from build123d import *

# Parameters (mm, degrees)
SKETCH_1_R          = 1.6
SKETCH_1_R_2        = 3.05
SKETCH_1_W          = 1.5
SKETCH_1_H          = 1.949874371
EXTRUDE_1_DEPTH     = 11
SKETCH_2_R          = 1.65
CUT_EXTRUDE_3_DEPTH = 21.223748416


with BuildPart() as part:
    # Sketch 1 → Extrude 1 (new body)
    # profile 1 of 23: a face of its own
    with BuildSketch(Plane.XY):
        with BuildLine():
            Line((-0.75, 9.971835338), (-0.75, 12))
            Line((-0.75, 12), (-1, 9.949874371))
            ThreePointArc((-1, 9.949874371), (-0.875068895, 9.961639144), (-0.75, 9.971835338))
        make_face()
    # profile 2 of 23: a face of its own
    with BuildSketch(Plane.XY):
        with BuildLine():
            Line((0.75, 12), (-0.75, 12))
            Line((-0.75, 12), (-0.75, 9.971835338))
            ThreePointArc((-0.75, 9.971835338), (0, 10), (0.75, 9.971835338))
            Line((0.75, 9.971835338), (0.75, 12))
        make_face()
    # profile 3 of 23: a face of its own
    with BuildSketch(Plane.XY):
        with BuildLine():
            ThreePointArc((-0.75, 9.971835338), (-0.875068895, 9.961639144), (-1, 9.949874371))
            Line((-1, 9.949874371), (-0.75, 9.949874371))
            Line((-0.75, 9.949874371), (-0.75, 9.971835338))
        make_face()
    # profile 4 of 23: a face of its own
    with BuildSketch(Plane.XY):
        with BuildLine():
            Line((-0.75, 9.949874371), (-1, 9.949874371))
            ThreePointArc((-1, 9.949874371), (-1.95090322, 9.807852804), (-2.883772543, 9.575168715))
            ThreePointArc((-2.883772543, 9.575168715), (-3.826834324, 9.238795325), (-4.731531608, 8.80980185))
            ThreePointArc((-4.731531608, 8.80980185), (-5.55570233, 8.314696123), (-6.328516859, 7.742730421))
            ThreePointArc((-6.328516859, 7.742730421), (-7.071067812, 7.071067812), (-7.742730421, 6.328516859))
            ThreePointArc((-7.742730421, 6.328516859), (-8.314696123, 5.55570233), (-8.80980185, 4.731531608))
            ThreePointArc((-8.80980185, 4.731531608), (-9.238795325, 3.826834324), (-9.575168715, 2.883772543))
            ThreePointArc((-9.575168715, 2.883772543), (-9.807852804, 1.95090322), (-9.949874371, 1))
            ThreePointArc((-9.949874371, 1), (-10, 0), (-9.949874371, -1))
            ThreePointArc((-9.949874371, -1), (-9.807852804, -1.95090322), (-9.575168715, -2.883772543))
            ThreePointArc((-9.575168715, -2.883772543), (-9.238795325, -3.826834324), (-8.80980185, -4.731531608))
            ThreePointArc((-8.80980185, -4.731531608), (-8.314696123, -5.55570233), (-7.742730421, -6.328516859))
            ThreePointArc((-7.742730421, -6.328516859), (-7.071067812, -7.071067812), (-6.328516859, -7.742730421))
            ThreePointArc((-6.328516859, -7.742730421), (-5.55570233, -8.314696123), (-4.731531608, -8.80980185))
            ThreePointArc((-4.731531608, -8.80980185), (-3.826834324, -9.238795325), (-2.883772543, -9.575168715))
            ThreePointArc((-2.883772543, -9.575168715), (-1.95090322, -9.807852804), (-1, -9.949874371))
            ThreePointArc((-1, -9.949874371), (0, -10), (1, -9.949874371))
            ThreePointArc((1, -9.949874371), (1.95090322, -9.807852804), (2.883772543, -9.575168715))
            ThreePointArc((2.883772543, -9.575168715), (3.826834324, -9.238795325), (4.731531608, -8.80980185))
            ThreePointArc((4.731531608, -8.80980185), (5.55570233, -8.314696123), (6.328516859, -7.742730421))
            ThreePointArc((6.328516859, -7.742730421), (7.071067812, -7.071067812), (7.742730421, -6.328516859))
            ThreePointArc((7.742730421, -6.328516859), (8.314696123, -5.55570233), (8.80980185, -4.731531608))
            ThreePointArc((8.80980185, -4.731531608), (9.238795325, -3.826834324), (9.575168715, -2.883772543))
            ThreePointArc((9.575168715, -2.883772543), (9.807852804, -1.95090322), (9.949874371, -1))
            ThreePointArc((9.949874371, -1), (9.987460731, -0.500627751), (10, 0))
            ThreePointArc((10, 0), (9.987460731, 0.500627751), (9.949874371, 1))
            ThreePointArc((9.949874371, 1), (9.807852804, 1.95090322), (9.575168715, 2.883772543))
            ThreePointArc((9.575168715, 2.883772543), (9.238795325, 3.826834324), (8.80980185, 4.731531608))
            ThreePointArc((8.80980185, 4.731531608), (8.314696123, 5.55570233), (7.742730421, 6.328516859))
            ThreePointArc((7.742730421, 6.328516859), (7.071067812, 7.071067812), (6.328516859, 7.742730421))
            ThreePointArc((6.328516859, 7.742730421), (5.55570233, 8.314696123), (4.731531608, 8.80980185))
            ThreePointArc((4.731531608, 8.80980185), (3.826834324, 9.238795325), (2.883772543, 9.575168715))
            ThreePointArc((2.883772543, 9.575168715), (1.95090322, 9.807852804), (1, 9.949874371))
            Line((1, 9.949874371), (0.75, 9.949874371))
            Line((0.75, 9.949874371), (0.75, 8))
            Line((0.75, 8), (-0.75, 8))
            Line((-0.75, 8), (-0.75, 9.949874371))
        make_face()
        with Locations((0, -6.363961031)):
            Circle(SKETCH_1_R, mode=Mode.SUBTRACT)
        with Locations((-6.363961031, 0)):
            Circle(SKETCH_1_R, mode=Mode.SUBTRACT)
        Circle(SKETCH_1_R_2, mode=Mode.SUBTRACT)
        with Locations((6.363961031, 0)):
            Circle(SKETCH_1_R, mode=Mode.SUBTRACT)
        with Locations((0, 6.363961031)):
            Circle(SKETCH_1_R, mode=Mode.SUBTRACT)
    # profile 5 of 23: a face of its own
    with BuildSketch(Plane.XY):
        with BuildLine():
            Line((1, 9.949874371), (0.75, 12))
            Line((0.75, 12), (0.75, 9.971835338))
            ThreePointArc((0.75, 9.971835338), (0.875068895, 9.961639144), (1, 9.949874371))
        make_face()
    # profile 6 of 23: a face of its own
    with BuildSketch(Plane.XY):
        with BuildLine():
            ThreePointArc((0.75, 9.971835338), (0, 10), (-0.75, 9.971835338))
            Line((-0.75, 9.971835338), (-0.75, 9.949874371))
            Line((-0.75, 9.949874371), (0.75, 9.949874371))
            Line((0.75, 9.949874371), (0.75, 9.971835338))
        make_face()
    # profile 7 of 23: a face of its own
    with BuildSketch(Plane.XY):
        with Locations((0, 8.974937185)):
            Rectangle(SKETCH_1_W, SKETCH_1_H)
    # profile 8 of 23: a face of its own
    with BuildSketch(Plane.XY):
        with BuildLine():
            ThreePointArc((-4.731531608, 8.80980185), (-3.826834324, 9.238795325), (-2.883772543, 9.575168715))
            Line((-2.883772543, 9.575168715), (-3.899291539, 11.373566964))
            Line((-3.899291539, 11.373566964), (-5.285110838, 10.799541816))
            Line((-5.285110838, 10.799541816), (-4.731531608, 8.80980185))
        make_face()
    # profile 9 of 23: a face of its own
    with BuildSketch(Plane.XY):
        with BuildLine():
            ThreePointArc((1, 9.949874371), (0.875068895, 9.961639144), (0.75, 9.971835338))
            Line((0.75, 9.971835338), (0.75, 9.949874371))
            Line((0.75, 9.949874371), (1, 9.949874371))
        make_face()
    # profile 10 of 23: a face of its own
    with BuildSketch(Plane.XY):
        with BuildLine():
            Line((3.899291539, 11.373566964), (2.883772543, 9.575168715))
            ThreePointArc((2.883772543, 9.575168715), (3.826834324, 9.238795325), (4.731531608, 8.80980185))
            Line((4.731531608, 8.80980185), (5.285110838, 10.799541816))
            Line((5.285110838, 10.799541816), (3.899291539, 11.373566964))
        make_face()
    # profile 11 of 23: a face of its own
    with BuildSketch(Plane.XY):
        with BuildLine():
            ThreePointArc((-7.742730421, 6.328516859), (-7.071067812, 7.071067812), (-6.328516859, 7.742730421))
            Line((-6.328516859, 7.742730421), (-7.954951288, 9.01561146))
            Line((-7.954951288, 9.01561146), (-9.01561146, 7.954951288))
            Line((-9.01561146, 7.954951288), (-7.742730421, 6.328516859))
        make_face()
    # profile 12 of 23: a face of its own
    with BuildSketch(Plane.XY):
        with BuildLine():
            Line((7.954951288, 9.01561146), (6.328516859, 7.742730421))
            ThreePointArc((6.328516859, 7.742730421), (7.071067812, 7.071067812), (7.742730421, 6.328516859))
            Line((7.742730421, 6.328516859), (9.01561146, 7.954951288))
            Line((9.01561146, 7.954951288), (7.954951288, 9.01561146))
        make_face()
    # profile 13 of 23: a face of its own
    with BuildSketch(Plane.XY):
        with BuildLine():
            ThreePointArc((-9.575168715, 2.883772543), (-9.238795325, 3.826834324), (-8.80980185, 4.731531608))
            Line((-8.80980185, 4.731531608), (-10.799541816, 5.285110838))
            Line((-10.799541816, 5.285110838), (-11.373566964, 3.899291539))
            Line((-11.373566964, 3.899291539), (-9.575168715, 2.883772543))
        make_face()
    # profile 14 of 23: a face of its own
    with BuildSketch(Plane.XY):
        with BuildLine():
            Line((10.799541816, 5.285110838), (8.80980185, 4.731531608))
            ThreePointArc((8.80980185, 4.731531608), (9.238795325, 3.826834324), (9.575168715, 2.883772543))
            Line((9.575168715, 2.883772543), (11.373566964, 3.899291539))
            Line((11.373566964, 3.899291539), (10.799541816, 5.285110838))
        make_face()
    # profile 15 of 23: a face of its own
    with BuildSketch(Plane.XY):
        with BuildLine():
            ThreePointArc((-9.949874371, -1), (-10, 0), (-9.949874371, 1))
            Line((-9.949874371, 1), (-12, 0.75))
            Line((-12, 0.75), (-12, -0.75))
            Line((-12, -0.75), (-9.949874371, -1))
        make_face()
    # profile 16 of 23: a face of its own
    with BuildSketch(Plane.XY):
        with BuildLine():
            Line((12, 0.75), (9.949874371, 1))
            ThreePointArc((9.949874371, 1), (9.987460731, 0.500627751), (10, 0))
            ThreePointArc((10, 0), (9.987460731, -0.500627751), (9.949874371, -1))
            Line((9.949874371, -1), (12, -0.75))
            Line((12, -0.75), (12, 0.75))
        make_face()
    # profile 17 of 23: a face of its own
    with BuildSketch(Plane.XY):
        with BuildLine():
            ThreePointArc((-8.80980185, -4.731531608), (-9.238795325, -3.826834324), (-9.575168715, -2.883772543))
            Line((-9.575168715, -2.883772543), (-11.373566964, -3.899291539))
            Line((-11.373566964, -3.899291539), (-10.799541816, -5.285110838))
            Line((-10.799541816, -5.285110838), (-8.80980185, -4.731531608))
        make_face()
    # profile 18 of 23: a face of its own
    with BuildSketch(Plane.XY):
        with BuildLine():
            ThreePointArc((-6.328516859, -7.742730421), (-7.071067812, -7.071067812), (-7.742730421, -6.328516859))
            Line((-7.742730421, -6.328516859), (-9.01561146, -7.954951288))
            Line((-9.01561146, -7.954951288), (-7.954951288, -9.01561146))
            Line((-7.954951288, -9.01561146), (-6.328516859, -7.742730421))
        make_face()
    # profile 19 of 23: a face of its own
    with BuildSketch(Plane.XY):
        with BuildLine():
            Line((11.373566964, -3.899291539), (9.575168715, -2.883772543))
            ThreePointArc((9.575168715, -2.883772543), (9.238795325, -3.826834324), (8.80980185, -4.731531608))
            Line((8.80980185, -4.731531608), (10.799541816, -5.285110838))
            Line((10.799541816, -5.285110838), (11.373566964, -3.899291539))
        make_face()
    # profile 20 of 23: a face of its own
    with BuildSketch(Plane.XY):
        with BuildLine():
            ThreePointArc((-2.883772543, -9.575168715), (-3.826834324, -9.238795325), (-4.731531608, -8.80980185))
            Line((-4.731531608, -8.80980185), (-5.285110838, -10.799541816))
            Line((-5.285110838, -10.799541816), (-3.899291539, -11.373566964))
            Line((-3.899291539, -11.373566964), (-2.883772543, -9.575168715))
        make_face()
    # profile 21 of 23: a face of its own
    with BuildSketch(Plane.XY):
        with BuildLine():
            Line((9.01561146, -7.954951288), (7.742730421, -6.328516859))
            ThreePointArc((7.742730421, -6.328516859), (7.071067812, -7.071067812), (6.328516859, -7.742730421))
            Line((6.328516859, -7.742730421), (7.954951288, -9.01561146))
            Line((7.954951288, -9.01561146), (9.01561146, -7.954951288))
        make_face()
    # profile 22 of 23: a face of its own
    with BuildSketch(Plane.XY):
        with BuildLine():
            ThreePointArc((1, -9.949874371), (0, -10), (-1, -9.949874371))
            Line((-1, -9.949874371), (-0.75, -12))
            Line((-0.75, -12), (0.75, -12))
            Line((0.75, -12), (1, -9.949874371))
        make_face()
    # profile 23 of 23: a face of its own
    with BuildSketch(Plane.XY):
        with BuildLine():
            Line((5.285110838, -10.799541816), (4.731531608, -8.80980185))
            ThreePointArc((4.731531608, -8.80980185), (3.826834324, -9.238795325), (2.883772543, -9.575168715))
            Line((2.883772543, -9.575168715), (3.899291539, -11.373566964))
            Line((3.899291539, -11.373566964), (5.285110838, -10.799541816))
        make_face()
    extrude(amount=EXTRUDE_1_DEPTH)

    # Sketch 2 → Cut-Extrude 3 (cut, through all)
    with BuildSketch(Plane(origin=(0, 0, 0), x_dir=(0, 0, -1), z_dir=(0.8314696123025446, -0.5555702330196034, 0))):
        with Locations(Location((-5.5, 0, 0), (0, 0, 90))):
            Circle(SKETCH_2_R)
    extrude(amount=-CUT_EXTRUDE_3_DEPTH, mode=Mode.SUBTRACT)


solid = part.part
The model under review builds one solid part; all positions refer to its coordinate system, in mm. A direction names the side the tool comes from. Give positions to 0.01 mm unless a question says otherwise; leave off trailing zeros. Write each loop counter-clockwise with the first axis right and the second up, starting at its lowest first coordinate (ties: lowest second). Pieces come first, ordered by that corner, then holes. Notation, with made-up numbers: M 72.25,11 L 93.25,11 A18 cw 93.25,35 Z; hole C -28,16.5 d3. An arc over 180 degrees is marked long. One line per question, with ' | ' between items. Start each with the question number.
Item 1: We need section C-C on x = 6.75. Write out the cut boundary in (y, z).
Item 2: Draft analysis for pull direction X (two halves, no side actions). For faces 1 (the flat face through (8.37, 7.13, 5.42)), 2 (the cylindrical face through (-8, -6, 5)), 3 (the flat face through (-8.48, 8.49, 5.42)), state which applies: released by +X, released by -X, zero draft, split by the parting line, or undercut.
Item 3: Wall thickness on line 1 (Y direction, x = 0, z = 7.5); line 2 (Y direction, x = 0.25, z = 7); line 3 (Y direction, x = 11, z = 0.75): over which ranges is each line inside the solid? List them lowest first. Write a range as from..to.
Item 4: For faces 4 (the flat face through (7.13, -8.37, 5.42)), 5 (the cylindrical face through (-8, 6, 9)), 6 (the cylindrical face through (2, 9.8, 5.4)), 7 (the cylindrical face through (9.81, 1.94, 5.42)), list the 3-axis set-ups (+Z, -Z, +X, -X, +Y, -Y) from which the entire face can be reached by the end or side of a thin tool; tool diameter is ignored.
Item 5: We need section D-D on z = 1.75. Give the number of separate pieces and of enclosed holes in the cut face, plus the area to 3 significant figures.
Item 6: We need section A-A on x = 0. Write out the cut boundary in (y, z).
Item 7: We need section B-B on x = 10.5. Write out the cut boundary in (y, z).
Item 8: For pin 1 (3 mm diameter, centred on y = -4, z = 3.5, fed in from -X); pin 2 (1 mm diameter, centred on x = -8, z = 9.5, fed in from +Y); pin 3 (1.5 mm diameter, centred on y = 3, z = 7.5, fed in from +X), all flat-tipped, find the tip position at first contact; note any pin that passes through.
Results found:
1) outline: M -8.07,0 L -1.55,0 L -1.55,11 L -8.07,11 Z; M 1.55,0 L 8.07,0 L 8.07,11 L 1.55,11 Z
2) face 1: released by +X | face 2: undercut | face 3: released by -X
3) line 1: y = -12..-7.96, -4.76..-3.05, 3.05..4.76, 7.96..12 | line 2: y = -12..-7.94, -4.78..-3.04, 3.04..4.78, 7.94..12 | line 3: y = -4.8..-3.69, -0.87..0.87, 3.69..4.8
4) face 4: +Z, -Z, -Y | face 5: +Z, -Z | face 6: +Z, -Z, +Y | face 7: +Z, -Z, +X
5) separate pieces: 1 | enclosed holes: 5 | area: 309 mm2
6) outline: M -12,0 L -7.96,0 L -7.96,11 L -12,11 Z; M -4.76,0 L -3.05,0 L -3.05,11 L -4.76,11 Z; M 3.05,0 L 4.76,0 L 4.76,11 L 3.05,11 Z; M 7.96,0 L 12,0 L 12,11 L 7.96,11 Z
7) outline: M -5.2,0 L -3.41,0 L -3.41,11 L -5.2,11 Z; M -0.93,0 L 0.93,0 L 0.93,11 L -0.93,11 Z; M 3.41,0 L 5.2,0 L 5.2,11 L 3.41,11 Z
8) pin 1: stops at x = -11.37 | pin 2: stops at y = 9.02 | pin 3: stops at x = 11.11
